Build history of the part. All positions in model axes, mm. Give positions to 0.01 mm unless a question says otherwise; leave off trailing zeros. Order: outer loops, then holes, each group sorted by start corner. A loop starts at its lowest first (then second) coordinate and runs counter-clockwise, first axis right, second up. Notation, with made-up numbers: (45, -3) - (91, -3) arc R32 cw to (91, 28) - close; hole circle Ø11 at (28.25, 18.25). An arc over 180 degrees is marked (long way). Use a Markdown table: item, result. Add a question column.
(1) Flat gauge pins, fed straight in: pin 1 (2 mm diameter, centred on x = 17.5, z = 1.5, fed in from +Y); pin 2 (2 mm diameter, centred on x = -7.5, z = 1, fed in from +Y). Where does each tip first touch, or does it go through?
(2) Slice it at A-A (z = 2.65). Write the cut outline in (x, y), then the cut area to 3 significant figures.
(3) Wall check: line 1 (X direction, y = 0, z = 2.6); line 2 (X direction, y = 0, z = 0.7); line 3 (Y direction, x = 0, z = 1.2). Give the ranges that are in metal, low to high.
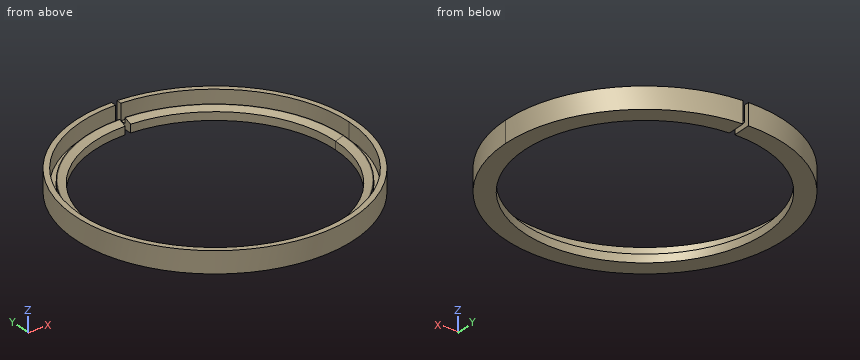
from build123d import *

# Parameters (mm, degrees)
F0_R     = 25.9
F0_R_2   = 22.4
F1_DEPTH = 2
F2_R     = 25.9
F2_R_2   = 24.9
F3_DEPTH = 2
F4_W     = 1
F4_H     = 10
F5_DEPTH = 25
F6_R     = 24.9
F6_R_2   = 23.9
F7_DEPTH = 1
F8_SIZE2 = 1.373739
F8_SIZE  = 0.5


with BuildPart() as f1:
    # F0 (on Top) → F1 (new body)
    with BuildSketch(Plane.XY):
        Circle(F0_R)
        Circle(F0_R_2, mode=Mode.SUBTRACT)
    extrude(amount=F1_DEPTH)

    # F2 (on face) → F3 (join)
    with BuildSketch(Plane.XY.offset(2)):
        Circle(F2_R)
        Circle(F2_R_2, mode=Mode.SUBTRACT)
    extrude(amount=F3_DEPTH)

    # F4 (on face) → F5 (cut)
    with BuildSketch(Plane(origin=(0, 0, 0), x_dir=(1, 0, 0), z_dir=(0, 0, -1))):
        with Locations((0, -25)):
            Rectangle(F4_W, F4_H)
    extrude(amount=-F5_DEPTH, mode=Mode.SUBTRACT)

    # F6 (on face) → F7 (cut)
    with BuildSketch(Plane.XY.offset(2)):
        Circle(F6_R)
        Circle(F6_R_2, mode=Mode.SUBTRACT)
    extrude(amount=-F7_DEPTH, mode=Mode.SUBTRACT)

    # F8
    f8_edges = [f1.edges().sort_by_distance(p)[0] for p in [
        (-15.661418, -16.014993, 2),
    ]]
    chamfer(f8_edges, length=F8_SIZE, length2=F8_SIZE2)


solid = f1.part
Solution:
| question | item | result |
|---|---|---|
| 1 | pin 1 | y = 19.96 |
| 1 | pin 2 | y = 25.07 |
| 2 | outline | (-0.5, 24.89) - (-0.5, 25.9) arc R25.9 ccw (long way) to (0.5, 25.9) - (0.5, 24.89) arc R24.9 cw (long way) to start |
| 2 | area | 159 mm2 |
| 3 | line 1 | -25.9 to -24.9, 24.9 to 25.9 |
| 3 | line 2 | -25.9 to -22.4, 22.4 to 25.9 |
| 3 | line 3 | -25.9 to -24.9, -23.9 to -22.4 |
